from build123d import *

# Parameters (mm, degrees)
SKETCH1_W           = 65
SKETCH1_H           = 87.5
SKETCH1_R           = 2.75
BOSS_EXTRUDE1_DEPTH = 10
FILLET1_R           = 10


with BuildPart() as part:
    # Sketch1 → Boss-Extrude1 (new body)
    with BuildSketch(Plane.XY):
        Rectangle(SKETCH1_W, SKETCH1_H)
        with Locations((-15, 36.25)):
            Circle(SKETCH1_R, mode=Mode.SUBTRACT)
        with Locations((0, 36.25)):
            Circle(SKETCH1_R, mode=Mode.SUBTRACT)
        with Locations((15, 36.25)):
            Circle(SKETCH1_R, mode=Mode.SUBTRACT)
    extrude(amount=BOSS_EXTRUDE1_DEPTH)

    # Fillet1
    fillet1_edges = [part.edges().sort_by_distance(p)[0] for p in [
        (-32.5, 43.75, 5),
        (32.5, 43.75, 5),
        (32.5, -43.75, 5),
        (-32.5, -43.75, 5),
    ]]
    fillet(fillet1_edges, radius=FILLET1_R)


solid = part.part
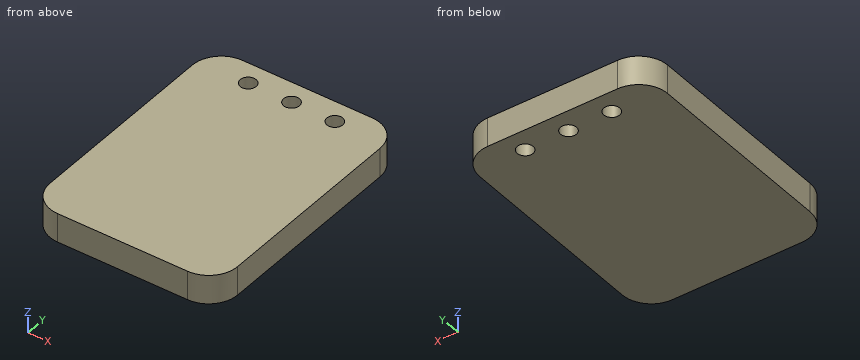
For this review, take the finished solid that the model builds, in its own axes (mm). Give positions to 0.01 mm unless a question says otherwise; leave off trailing zeros. Loops run counter-clockwise (first coordinate to the right, second up) from the corner with the lowest first, then second, coordinate; pieces in that order, holes last. Notation, with made-up numbers: M -5.5,8.5 L 49.5,8.5 A17 ccw 49.5,19.5 Z; hole C 58,85.25 d11. An arc over 180 degrees is marked long. Put each result on its own line as item: value. Start each with the question number.
(1) For pin 1 (1 mm diameter, centred on x = -4.5, y = -4.5, fed in from -Z); pin 2 (1 mm diameter, centred on x = 25, z = 4.5, fed in from +Y), all flat-tipped, find the tip position at first contact; note any pin that passes through.
(2) Add section A-A, the plane x = 0. Write out the cut boundary in (y, z).
(3) Add section C-C, the plane y = 36.25. Write out the cut boundary in (x, z), then the cut area to 3 significant figures.
(4) Add section B-B, the plane z = 7.25. Write out the cut boundary in (x, y).
(5) Wall thickness on L1, parallel to Y at x = -15, z = 7.5; L2, parallel to Y at x = 1.5, z = 7.5; L3, parallel to Y at x = 27, z = 6: over which ranges is each line inside the solid? List them lowest first.
Result:
1. pin 1: stops at z = 0
1. pin 2: stops at y = 43.55
2. outline: M -43.75,0 L 33.5,0 L 33.5,10 L -43.75,10 Z; M 39,0 L 43.75,0 L 43.75,10 L 39,10 Z
3. outline: M -32.18,0 L -17.75,0 L -17.75,10 L -32.18,10 Z; M -12.25,0 L -2.75,0 L -2.75,10 L -12.25,10 Z; M 2.75,0 L 12.25,0 L 12.25,10 L 2.75,10 Z; M 17.75,0 L 32.18,0 L 32.18,10 L 17.75,10 Z
3. area: 479 mm^2
4. outline: M -32.5,-33.75 A10 ccw -22.5,-43.75 L 22.5,-43.75 A10 ccw 32.5,-33.75 L 32.5,33.75 A10 ccw 22.5,43.75 L -22.5,43.75 A10 ccw -32.5,33.75 Z; hole C -15,36.25 d5.5; hole C 0,36.25 d5.5; hole C 15,36.25 d5.5
5. L1: y = -43.75 to 33.5, 39 to 43.75
5. L2: y = -43.75 to 33.95, 38.55 to 43.75
5. L3: y = -42.68 to 42.68
